Input: part model. Units: mm. Frame: model coordinates. Face numbers are marked on the shaded views. A direction names the side the tool comes from. Round coordinates to 2 decimals unless told otherwise and drop trailing zeros. Order: outer loops, then holes, each group sorted by start corner. A loop starts at its lowest first (then second) coordinate and runs counter-clockwise, first axis right, second up. Notation, with made-up numbers: (3.25, 10) -> (41.25, 10) arc R12 ccw to (41.25, 19) -> close; hole circle Ø5 at (68.5, -5.75). An arc over 180 degrees is marked (long way). Answer as CSV lines item,"result". Start each with the question number.
1) Mould query, pull axis Z, two halves, no side actions, for the marked faces 5, 6 and 7. Classes: +Z half, -Z half, draft (parallel to the pull), parting line (faces both ways), or undercut.
2) Section query A-A, the plane y = -501. Output: boundary loops of the cut face in (x, z), and give its area (3 significant figures).
3) Section query C-C, the plane z = 888. Output: boundary loops of the cut face in (x, y).
4) Access query for the marked faces 1, 2, 3 and 4. Directions: +Z, -Z, +X, -X, +Y, -Y. A direction counts if a zero-diameter tool reaches every point of the face in a straight line with its end or side. Return the directions, or none.
5) Line query: L1, parallel to Z at x = 274.5, y = -441; L2, parallel to X at y = -557, z = 945.5; L3, parallel to Y at x = 36, z = 474. Output: solid intervals per line, ascending.
6) Section query B-B, the plane x = 318.5. Output: boundary loops of the cut face in (y, z), and give its area (3 significant figures).
7) First-contact query: P1, Ø3, axis at x = 56.5, z = 426.5, coming from the -Y side; P2, Ø12, axis at x = 60, z = 567, coming from the +Y side; P3, Ø4, axis at y = -114, z = 332, coming from the +X side. Flat tips, straight axial feed; report the tip coordinate or a pass-through.
```python
from build123d import *

# Parameters (mm, degrees)
F0_W     = 457.2
F0_H     = 673.1
F1_DEPTH = 1289.05
F2_W     = 460.375
F2_H     = 676.275
F2_W_2   = 457.2
F2_H_2   = 673.1
F3_DEPTH = 31.75
F4_W     = 419.1
F4_H     = 292.1
F5_DEPTH = 666.75


with BuildPart() as f1:
    # F0 (on Top) → F1 (new body)
    with BuildSketch(Plane.XY):
        with Locations((228.6, -336.55)):
            Rectangle(F0_W, F0_H)
    extrude(amount=F1_DEPTH)

    # F2 (on face) → F3 (join)
    with BuildSketch(Plane.XY.offset(1289.05)):
        with Locations((228.6, -336.55)):
            Rectangle(F2_W, F2_H)
        with Locations((228.6, -336.55)):
            Rectangle(F2_W_2, F2_H_2, mode=Mode.SUBTRACT)
        with Locations((228.6, -336.55)):
            Rectangle(F2_W_2, F2_H_2)
    extrude(amount=F3_DEPTH)

    # F4 (on face) → F5 (cut)
    with BuildSketch(Plane.XZ.offset(673.1)):
        with Locations((228.6, 1143)):
            Rectangle(F4_W, F4_H)
        with Locations((228.6, 838.2)):
            Rectangle(F4_W, F4_H)
        with Locations((228.6, 533.4)):
            Rectangle(F4_W, F4_H)
        with Locations((228.6, 228.6)):
            Rectangle(F4_W, F4_H)
    extrude(amount=-F5_DEPTH, mode=Mode.SUBTRACT)


solid = f1.part
```
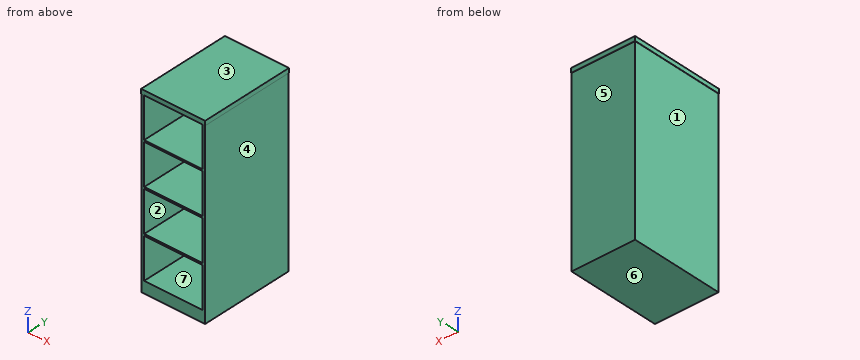
Findings:
1,face 5,"draft"
1,face 6,"-Z half"
1,face 7,"undercut"
2,outline,"(-1.59, 1289.05) -> (0, 1289.05) -> (0, 0) -> (457.2, 0) -> (457.2, 1289.05) -> (458.79, 1289.05) -> (458.79, 1320.8) -> (-1.59, 1320.8) -> close; hole (19.05, 82.55) -> (438.15, 82.55) -> (438.15, 374.65) -> (19.05, 374.65) -> close; hole (19.05, 387.35) -> (438.15, 387.35) -> (438.15, 679.45) -> (19.05, 679.45) -> close; hole (19.05, 692.15) -> (438.15, 692.15) -> (438.15, 984.25) -> (19.05, 984.25) -> close; hole (19.05, 996.95) -> (438.15, 996.95) -> (438.15, 1289.05) -> (19.05, 1289.05) -> close"
2,area,"114,000 mm^2"
3,outline,"(0, -673.1) -> (19.05, -673.1) -> (19.05, -6.35) -> (438.15, -6.35) -> (438.15, -673.1) -> (457.2, -673.1) -> (457.2, 0) -> (0, 0) -> close"
4,face 1,"-Z, -X, +Y, -Y"
4,face 2,"-Y"
4,face 3,"+Z, +X, -X, +Y, -Y"
4,face 4,"-Z, +X, +Y, -Y"
5,L1,"z = 0 to 82.55, 374.65 to 387.35, 679.45 to 692.15, 984.25 to 996.95, 1289.05 to 1320.8"
5,L2,"x = 0 to 19.05, 438.15 to 457.2"
5,L3,"y = -6.35 to 0"
6,outline,"(-674.69, 1289.05) -> (-6.35, 1289.05) -> (-6.35, 996.95) -> (-673.1, 996.95) -> (-673.1, 984.25) -> (-6.35, 984.25) -> (-6.35, 692.15) -> (-673.1, 692.15) -> (-673.1, 679.45) -> (-6.35, 679.45) -> (-6.35, 387.35) -> (-673.1, 387.35) -> (-673.1, 374.65) -> (-6.35, 374.65) -> (-6.35, 82.55) -> (-673.1, 82.55) -> (-673.1, 0) -> (0, 0) -> (0, 1289.05) -> (1.59, 1289.05) -> (1.59, 1320.8) -> (-674.69, 1320.8) -> close"
6,area,"110,000 mm^2"
7,P1,"stops at y = -6.35"
7,P2,"stops at y = 0"
7,P3,"stops at x = 457.2"
